from build123d import *

# Parameters (mm, degrees)
F0_W     = 304.8
F0_H     = 609.6
F1_DEPTH = 101.6
F2_W     = 609.6
F2_H     = 609.6
F3_DEPTH = 50.8
F4_W     = 304.8
F4_H     = 304.8
F5_DEPTH = 101.6


with BuildPart() as f1:
    # F0 (on Top) → F1 (new body)
    with BuildSketch(Plane.XY):
        Rectangle(F0_W, F0_H)
    extrude(amount=F1_DEPTH)

    # F2 (on Top) → F3 (join)
    with BuildSketch(Plane.XY):
        Rectangle(F2_W, F2_H)
    extrude(amount=-F3_DEPTH)

    # F4 (on face) → F5 (join)
    with BuildSketch(Plane.XY.offset(101.6)):
        Rectangle(F4_W, F4_H)
    extrude(amount=F5_DEPTH)


solid = f1.part
The listing builds one solid part. Answer for the finished solid, in the listing's coordinates (mm). A direction names the side the tool comes from. Coordinates: 2 decimals unless noted, no trailing zeros. Write each loop counter-clockwise with the first axis right and the second up, starting at its lowest first coordinate (ties: lowest second). Pieces come first, ordered by that corner, then holes. Notation, with made-up numbers: (-39, 54) - (14, 54) arc R5 ccw to (14, 58) - close; hole circle Ø1 at (69, 42). An arc over 180 degrees is marked (long way). Put each result on its own line as item: value.
1. The part is cut by section C-C on z = 8.5. Give the vertices of the cut face in (x, y).
Answer sheet:
outline: (-152.4, -304.8) - (152.4, -304.8) - (152.4, 304.8) - (-152.4, 304.8) - close
2. The part is cut by section A-A on y = 127. Give the vertices of the cut face in (x, z), plus the area to 3 significant figures.
Answer sheet:
outline: (-304.8, -50.8) - (304.8, -50.8) - (304.8, 0) - (152.4, 0) - (152.4, 203.2) - (-152.4, 203.2) - (-152.4, 0) - (-304.8, 0) - close
area: 92,900 mm^2
3. Flat-ended cylindrical pins translate along their axes: pin 1 Ø12 at (y, z) = (-110, 95) entering from -X; pin 2 Ø10 at (y, z) = (-134, 86) entering from +X; pin 3 Ø12 at (x, y) = (-229.5, 216) entering from +Z. Find the tip coordinate at first contact, or state that the pin passes through.
Answer sheet:
pin 1: stops at x = -152.4
pin 2: stops at x = 152.4
pin 3: stops at z = 0
4. Find the intervals of material crossed by line 1 along X through (y, z) = (-59.5, 175.5); line 2 along Z through (x, y) = (272.5, 53); line 3 along Z through (x, y) = (27, 202), in increasing order. Write a range as from..to.
Answer sheet:
line 1: x = -152.4..152.4
line 2: z = -50.8..0
line 3: z = -50.8..101.6
5. The part is cut by section B-B on x = 92. Give the vertices of the cut face in (y, z).
Answer sheet:
outline: (-304.8, -50.8) - (304.8, -50.8) - (304.8, 101.6) - (152.4, 101.6) - (152.4, 203.2) - (-152.4, 203.2) - (-152.4, 101.6) - (-304.8, 101.6) - close
6. The part is cut by section D-D on x = -251. Give the vertices of the cut face in (y, z), plus the area to 3 significant figures.
Answer sheet:
outline: (-304.8, -50.8) - (304.8, -50.8) - (304.8, 0) - (-304.8, 0) - close
area: 31,000 mm^2
7. A tool of negligible diameter and unlimited length cuts with its end or side. For faces 1 (the face through (152.4, -4, 78)), 2 (the face through (-2, -228, 101.6)), 3 (the face through (-230, 4, 0)), 4 (the face through (-2, 230, 101.6)), from which of +Z, -Z, +X, -X, +Y, -Y can it reach the whole face along a straight path? Write none if from no direction.
Answer sheet:
face 1: +Z, +X, +Y, -Y
face 2: +Z, +X, -X, -Y
face 3: +Z, -X, +Y, -Y
face 4: +Z, +X, -X, +Y
